Autodesk Inventor part; units mm, degrees
ref_plane "Work Plane1" through (0, 0, 0) normal (0, 0, 1) x (1, 0, 0)
ref_plane "YZ Plane" through (0, 0, 0) normal (1, 0, 0) x (0, 1, 0)
ref_plane "XZ Plane" through (0, 0, 0) normal (0, 1, 0) x (-1, 0, 0)
ref_plane "Work Plane1" through (0, 0, 0) normal (0, 0, 1) x (1, 0, 0)
sketch "Sketch1" plane through (0, 0, 0) normal (0, 0, 1) x (1, 0, 0)
  circle A0 centre (22.2, -27.45) radius 1.5
  circle A1 centre (58.6, -27.45) radius 1.5
  circle A2 centre (22.2, 9.15) radius 1.5
  circle A3 centre (58.6, 9.15) radius 1.5
  line L0 (15.5, 16.5) -> (15.5, -25.3)
  line L1 (19.5, -29.3) -> (61, -29.3)
  line L2 (61, 20.5) -> (19.5, 20.5)
  line L3 (64.8607, 14) -> (64.8607, -18)
  line L4 (65.75, -18) -> (65.75, 14)
  line L5 (65.75, -33.3) -> (51.75, -33.3)
  line L6 (51.75, -33.3) -> (51.75, -21.8024)
  line L7 (55.4368, -18.3) -> (65.75, -18.3)
  line L8 (65.75, -18.3) -> (65.75, -33.3)
  line L9 (15.5, -33.3) -> (29.5, -33.3)
  line L10 (29.5, -33.3) -> (29.5, -21.8024)
  line L11 (25.8132, -18.3) -> (15.5, -18.3)
  line L12 (15.5, -18.3) -> (15.5, -33.3)
  line L13 (15.5, 20.5697) -> (29.5, 20.5697)
  line L14 (29.5, 20.5697) -> (29.5, 9.0024)
  line L15 (25.8695, 5.5697) -> (15.5, 5.5697)
  line L16 (15.5, 5.5697) -> (15.5, 20.5697)
  line L17 (51.75, 20.5697) -> (65.75, 20.5697)
  line L18 (65.75, 20.5697) -> (65.75, 5.5697)
  line L19 (65.75, 5.5697) -> (55.3805, 5.5697)
  line L20 (51.75, 9.0024) -> (51.75, 20.5697)
  arc A4 (51.75, 9.0024) -> (29.5, 9.0024) centre (40.625, -6.4) ccw
  arc A5 (25.8695, 5.5697) -> (25.8132, -18.3) centre (40.625, -6.4) ccw
  arc A6 (29.5, -21.8024) -> (51.75, -21.8024) centre (40.625, -6.4) ccw
  arc A7 (55.4368, -18.3) -> (55.3805, 5.5697) centre (40.625, -6.4) ccw
  line L21 (65.75, 20.5697) -> (65.75, 5.5697)
  line L22 (65.75, -18.3) -> (65.75, -33.3)
  line L23 (15.5, 20.5697) -> (29.5, 20.5697)
  line L24 (51.75, 20.5697) -> (65.75, 20.5697)
  line L25 (15.5, -33.3) -> (15.5, -18.3)
  line L26 (15.5, 5.5697) -> (15.5, 20.5697)
  point P0 (0, 0)
  point P1 (40.25, 20.5)
  dimension "d10" = 50.25
  dimension "d13" = 26.9
extrude "Extrusion1" add sketch "Sketch1" along normal blind 2 contours L16 L13 L14 A4 L20 L17 L18 L4 L19 A7 L7 L8 L5 L6 A6 L10 L9 L12 L0 L11 A5 L15
fillet "Fillet1" radius 3 7 edges at (55.3805, 5.5697, 1) (29.5, -21.8024, 1) (25.8132, -18.3, 1) (29.5, 9.0024, 1) (55.4368, -18.3, 1) (25.8695, 5.5697, 1) (51.75, -21.8024, 1)
fillet "Fillet2" radius 3 12 edges at (15.5, 20.5697, 1) (15.5, 5.5697, 1) (29.5, 20.5697, 1) (51.75, 20.5697, 1) (65.75, 20.5697, 1) (65.75, -18.3, 1) (51.75, -33.3, 1) (15.5, -18.3, 1) (15.5, -33.3, 1) (29.5, -33.3, 1) (65.75, -33.3, 1) (65.75, 5.5697, 1)
sketch "Sketch2" plane through (0, 0, 2) normal (0, 0, 1) x (1, 0, 0)
  circle A0 centre (60.25, -23.1) radius 1.6
  circle A1 centre (20.25, -23.1) radius 1.6
  circle A2 centre (20.25, 16.9) radius 1.6
  circle A3 centre (60.25, 16.9) radius 1.6
  circle A4 centre (20.25, -23.1) radius 2.5
  circle A5 centre (60.25, 16.9) radius 2.5
  circle A6 centre (20.25, 16.9) radius 2.5
  circle A7 centre (60.25, -23.1) radius 2.5
  point P0 (0, 0)
  dimension "d17" = 5
  dimension "d18" = 5
  dimension "d19" = 5
  dimension "d20" = 5
extrude "Extrusion2" add sketch "Sketch2" along normal blind 26
fillet "Fillet3" radius 3 1 edges at (51.75, 9.0024, 1)
equation "\"d13\" = 0.5 * d11"
properties part number "soporteHBridge" material "ABS Plastic"
For this review, take the finished solid that the model builds, in its own axes (mm). A direction names the side the tool comes from. Round coordinates to 2 decimals unless told otherwise and drop trailing zeros. Write each loop counter-clockwise with the first axis right and the second up, starting at its lowest first coordinate (ties: lowest second). Pieces come first, ordered by that corner, then holes. Notation, with made-up numbers: (68, -2.5) -> (80, -2.5) arc R13 cw to (80, 13.5) -> close; hole circle Ø1 at (0.25, 75). An arc over 180 degrees is marked (long way). Use one line per item in the form item = value.
Q1. The part is to be moulded in two halves that separate along Y. For faces 1 (the flat face through (20, -25, 28)), 2 (the cylindrical face through (57.49, 8.14, 0.99)), 3 (the cylindrical face through (64.89, 19.67, 1.01)), 4 (the cylindrical face through (28.6, -32.44, 1.01)), say which applies: released by +Y, released by -Y, zero draft, split by the parting line, or undercut.
Resolved:
face_1 = zero draft
face_2 = undercut
face_3 = released by +Y
face_4 = released by -Y
Q2. Consider section C-C (x = 25). State the section outline as (y, z) points, then the cut area to 3 significant figures.
Resolved:
outline = (-33.3, 0) -> (20.57, 0) -> (20.57, 2) -> (-33.3, 2) -> close
area = 108 mm²
Q3. Machinability: for faces 5 (the cylindrical face through (61.776, -23.581, 14.818)), 6 (the cylindrical face through (52.61, -32.4, 1.01)), 7 (the cylindrical face through (58.208, -16.902, 1.014)), 8 (the cylindrical face through (16.36, 6.47, 1.01)), which of the approach directions +Z, -Z, +X, -X, +Y, -Y give a long, thin tool a straight path to every point of the face, cutting with its end or side? Answer none if there is none.
Resolved:
face_5 = +Z
face_6 = +Z, -Z, -Y
face_7 = +Z, -Z, +X
face_8 = +Z, -Z, -X
Q4. Consider section B-B (y = -23.1). State the section outline as (x, z) points, then the cut area to 3 significant figures.
Resolved:
outline = (15.5, 0) -> (65.75, 0) -> (65.75, 2) -> (62.75, 2) -> (62.75, 28) -> (61.85, 28) -> (61.85, 2) -> (58.65, 2) -> (58.65, 28) -> (57.75, 28) -> (57.75, 2) -> (22.75, 2) -> (22.75, 28) -> (21.85, 28) -> (21.85, 2) -> (18.65, 2) -> (18.65, 28) -> (17.75, 28) -> (17.75, 2) -> (15.5, 2) -> close
area = 194 mm²
Q5. Consider section A-A (y = 16.9). State the section outline as (x, z) points.
Resolved:
outline = (15.5, 0) -> (29.5, 0) -> (29.5, 2) -> (22.75, 2) -> (22.75, 28) -> (21.85, 28) -> (21.85, 2) -> (18.65, 2) -> (18.65, 28) -> (17.75, 28) -> (17.75, 2) -> (15.5, 2) -> close; (51.75, 0) -> (65.75, 0) -> (65.75, 2) -> (62.75, 2) -> (62.75, 28) -> (61.85, 28) -> (61.85, 2) -> (58.65, 2) -> (58.65, 28) -> (57.75, 28) -> (57.75, 2) -> (51.75, 2) -> close
Q6. To check wall thickness, follow probe 1 along Y at (x, z) = (20.25, 22.75); probe 2 along Z at (x, y) = (22, -9); probe 3 along X at (y, z) = (-6.5, 1.5). State the ranges of each line that lie inside material, in increasing order. Write a range as from..to.
Resolved:
probe_1 = -25.6..-24.7, -21.5..-20.6, 14.4..15.3, 18.5..19.4
probe_2 = 0..2
probe_3 = 21.63..59.62
Q7. Clearance check with a flat-ended pin moving along its axis: pin 1 Ø3.5 at (x, y) = (58.6, -27.45) entering from +Z. State where the tip first meets the part, or that it passes through.
Resolved:
pin_1 = 2
Q8. Consider section D-D (x = 50). State the section outline as (y, z) points.
Resolved:
outline = (-24.12, 0) -> (11.32, 0) -> (11.32, 2) -> (-24.12, 2) -> close
